Check sheet for the modelled part. Datum: model origin and axes. Units: mm. Give positions to 0.01 mm unless a question says otherwise; leave off trailing zeros. Loops run counter-clockwise (first coordinate to the right, second up) from the corner with the lowest first, then second, coordinate; pieces in that order, holes last. Notation, with made-up numbers: (15.5, -26) -> (28.5, -26) arc R30 cw to (28.5, -1) -> close; hole circle Ø4 at (87, -6). An arc over 180 degrees is marked (long way). Write each question's results on one line, items separated by ' | '. Start each with the question number.
1. Gauge pin test, flat end, axial feed: pin 1 Ø7 at (x, y) = (4042.18, 1222.59) entering from -Z. Record the tip position at first contact, or that the pin passes through.
2. Material ranges on L1, parallel to X at y = 1223, z = 1.8; L2, parallel to X at y = 1236, z = 0.65; L3, parallel to Y at x = 4041.5, z = 1.55, recorded low to high. Write a range as from..to.
3. Cross-section at B-B on y = 1225. Record the boundary of the cut face in (x, z), and give its area (3 significant figures).
4. Cross-section at A-A on x = 4023. Record the boundary of the cut face in (y, z) (3 decimals).
5. Mould release check, pull along X, two halves, no side actions. Record for faces 1 (the face through (4037.881, 1232.668, 0.986)), 2 (the face through (4013.58, 1262.62, 0.99)), 3 (the face through (4013, 1267.999, 1)), 4 (the face through (4049.036, 1225.911, 0.986)): +X half, -X half, draft (parallel to the pull), parting line (faces both ways), or undercut.
6. Cross-section at D-D on x = 4006. Record the boundary of the cut face in (y, z).
7. Cross-section at C-C on z = 1.2. Record the boundary of the cut face in (x, y), and give its area (3 significant figures).
from build123d import *

# Parameters (mm, degrees)
CROQUIS1_R              = 3.811830968
CROQUIS1_R_2            = 8.433713649
CROQUIS1_R_3            = 5.50644924
CROQUIS1_R_4            = 1
SALIENTE_EXTRUIR1_DEPTH = 2


with BuildPart() as part:
    # Croquis1 → Saliente-Extruir1 (new body)
    with BuildSketch(Plane.XY):
        with BuildLine():
            Line((4031.0864923, 1267.998645222), (3994.220839377, 1267.998645222))
            ThreePointArc((3994.220839377, 1267.998645222), (4029.544836626, 1223.835026243), (4073.293708821, 1187.998645222))
            ThreePointArc((4073.293708821, 1187.998645222), (4074.595594818, 1188.175999527), (4074.598031282, 1189.48990811))
            ThreePointArc((4074.598031282, 1189.48990811), (4048.728408118, 1226.464274325), (4031.0864923, 1267.998645222))
        make_face()
        with Locations((4042.182467754, 1222.589537582)):
            Circle(CROQUIS1_R, mode=Mode.SUBTRACT)
        with Locations((4021.504921686, 1251.374870701)):
            Circle(CROQUIS1_R_2, mode=Mode.SUBTRACT)
        with Locations((4032.794850615, 1234.777177731)):
            Circle(CROQUIS1_R_3, mode=Mode.SUBTRACT)
        with Locations((4012.653665839, 1262.998645222)):
            Circle(CROQUIS1_R_4, mode=Mode.SUBTRACT)
    extrude(amount=SALIENTE_EXTRUIR1_DEPTH)


solid = part.part
Geometry says:
1) pin 1: through
2) L1: 4030.37..4038.39, 4045.97..4050.69 | L2: 4018.24..4027.43, 4038.16..4043.75 | L3: 1212.46..1218.84, 1226.34..1240.72
3) outline: (4028.4, 0) -> (4039.23, 0) -> (4039.23, 2) -> (4028.4, 2) -> close; (4045.14, 0) -> (4049.55, 0) -> (4049.55, 2) -> (4045.14, 2) -> close | area: 30.5 mm^2
4) outline: (1230.693, 0) -> (1243.075, 0) -> (1243.075, 2) -> (1230.693, 2) -> close; (1259.675, 0) -> (1267.999, 0) -> (1267.999, 2) -> (1259.675, 2) -> close
5) face 1: undercut | face 2: undercut | face 3: draft | face 4: +X half
6) outline: (1251.07, 0) -> (1268, 0) -> (1268, 2) -> (1251.07, 2) -> close
7) outline: (3994.22, 1268) arc R269.99 ccw to (4073.29, 1188) arc R1 ccw to (4074.6, 1189.49) arc R216.47 cw to (4031.09, 1268) -> close; hole circle Ø2 at (4012.65, 1263); hole circle Ø16.87 at (4021.5, 1251.37); hole circle Ø11.01 at (4032.79, 1234.78); hole circle Ø7.62 at (4042.18, 1222.59) | area: 1,360 mm^2
